Check sheet for the modelled part. Datum: model origin and axes. Units: mm. Face numbers are marked on the shaded views. A direction names the side the tool comes from. Round coordinates to 2 decimals unless told otherwise and drop trailing zeros. Order: outer loops, then holes, each group sorted by start corner. A loop starts at its lowest first (then second) coordinate and runs counter-clockwise, first axis right, second up. Notation, with made-up numbers: (36.25, 45.25) -> (49.25, 45.25) arc R19 cw to (49.25, 77.25) -> close; hole circle Ø10 at (68.25, 73). An arc over 180 degrees is marked (long way). Use CSV: the item, a comma, the result in double quotes.
```python
from build123d import *

# Parameters (mm, degrees)
SKETCH1_W           = 42
SKETCH1_H           = 25
BOSS_EXTRUDE1_DEPTH = 3
SKETCH2_W           = 42
SKETCH2_H           = 17
BOSS_EXTRUDE2_DEPTH = 6
SKETCH4_W           = 42
SKETCH4_H           = 3
BOSS_EXTRUDE4_DEPTH = 3
FILLET2_R           = 2
SKETCH5_W           = 42
SKETCH5_H           = 3
BOSS_EXTRUDE5_DEPTH = 2
SKETCH7_W           = 42
SKETCH7_H           = 3
BOSS_EXTRUDE6_DEPTH = 20
BOSS_EXTRUDE7_DEPTH = 50
BOSS_EXTRUDE8_DEPTH = 13
CUT_EXTRUDE1_DEPTH  = 13
FILLET3_R           = 10


with BuildPart() as part:
    # Sketch1 → Boss-Extrude1 (new body)
    with BuildSketch(Plane(origin=(0, 0, 0), x_dir=(1, 0, 0), z_dir=(0, 1, 0))):
        Rectangle(SKETCH1_W, SKETCH1_H)
    extrude(amount=BOSS_EXTRUDE1_DEPTH)

    # Sketch2 → Boss-Extrude2 (add)
    with BuildSketch(Plane(origin=(0, 0, 0), x_dir=(1, 0, 0), z_dir=(0, 1, 0))):
        with Locations((0, 21)):
            Rectangle(SKETCH2_W, SKETCH2_H)
    extrude(amount=BOSS_EXTRUDE2_DEPTH)

    # Sketch4 → Boss-Extrude4 (add)
    with BuildSketch(Plane(origin=(0, 0, -29.5), x_dir=(-1, 0, 0), z_dir=(0, 0, -1))):
        with Locations((0, 4.5)):
            Rectangle(SKETCH4_W, SKETCH4_H)
    extrude(amount=BOSS_EXTRUDE4_DEPTH)

    # Fillet2
    fillet2_edges = [part.edges().sort_by_distance(p)[0] for p in [
        (0, 3, -29.5),
    ]]
    fillet(fillet2_edges, radius=FILLET2_R)

    # Sketch5 → Boss-Extrude5 (add)
    with BuildSketch(Plane(origin=(0, 0, -32.5), x_dir=(-1, 0, 0), z_dir=(0, 0, -1))):
        with Locations((0, 4.5)):
            Rectangle(SKETCH5_W, SKETCH5_H)
    extrude(amount=BOSS_EXTRUDE5_DEPTH)

    # Sketch7 → Boss-Extrude6 (add)
    with BuildSketch(Plane(origin=(0, 0, -34.5), x_dir=(-1, 0, 0), z_dir=(0, 0, -1))):
        with Locations((0, 4.5)):
            Rectangle(SKETCH7_W, SKETCH7_H)
    extrude(amount=BOSS_EXTRUDE6_DEPTH)

    # Sketch6 → Boss-Extrude7 (add)
    with BuildSketch(Plane(origin=(0, 6, 0), x_dir=(1, 0, 0), z_dir=(0, 1, 0))):
        Polygon((-21, 34.5), (-1, 34.5), (-1, 54.5), (1, 54.5), (1, 34.5), (21, 34.5), (21, 32.5), (1, 32.5), (1, 12.5), (-1, 12.5), (-1, 32.5), (-21, 32.5), align=None)
    extrude(amount=BOSS_EXTRUDE7_DEPTH)

    # Sketch9 → Boss-Extrude8 (add)
    with BuildSketch(Plane(origin=(0, 6, 0), x_dir=(1, 0, 0), z_dir=(0, 1, 0))):
        Polygon((-12, 34.5), (-1, 45.5), (-1, 34.5), align=None)
        Polygon((1, 34.5), (1, 45.5), (12, 34.5), align=None)
        Polygon((12, 32.5), (1, 32.5), (1, 21.5), align=None)
        Polygon((-1, 21.5), (-1, 32.5), (-12, 32.5), align=None)
    extrude(amount=BOSS_EXTRUDE8_DEPTH)

    # Sketch10 → Cut-Extrude1 (cut)
    with BuildSketch(Plane(origin=(0, 6, 0), x_dir=(1, 0, 0), z_dir=(0, 1, 0))):
        Polygon((1, 45.5), (1, 51.581118318), (18.081118318, 34.5), (12, 34.5), align=None)
        Polygon((-1, 45.5), (-1, 51.581118318), (-18.081118318, 34.5), (-12, 34.5), align=None)
        Polygon((-12, 32.5), (-1, 21.5), (-1, 15.418881682), (-18.081118318, 32.5), align=None)
        Polygon((1, 21.5), (1, 15.418881682), (18.081118318, 32.5), (12, 32.5), align=None)
    extrude(amount=-CUT_EXTRUDE1_DEPTH, mode=Mode.SUBTRACT)

    # Fillet3
    fillet3_edges = [part.edges().sort_by_distance(p)[0] for p in [
        (21, 4.5, -54.5),
        (-21, 4.5, -54.5),
    ]]
    fillet(fillet3_edges, radius=FILLET3_R)


solid = part.part
```
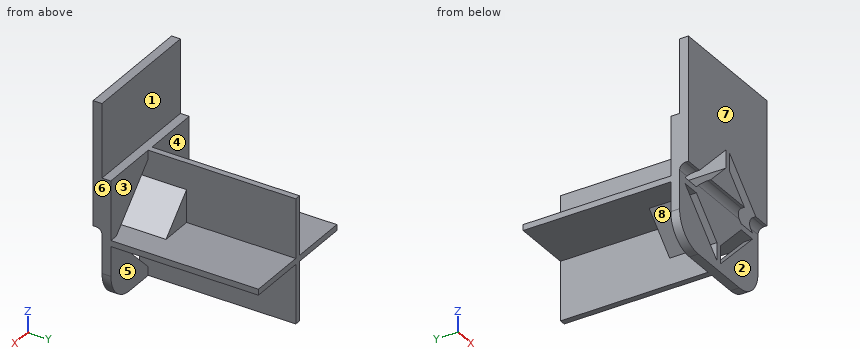
Q1. Scan lines: L1, parallel to X at y = 5, z = -16; L2, parallel to X at y = 2, z = -27.5; L3, parallel to Z at x = 4.5, y = 4. Record each from-to range of solid material in increasing order.
Result sheet:
L1,"x = -21 to -1.58, -1 to 1, 1.58 to 21"
L2,"x = -21 to -13.08, -7 to 7, 13.08 to 21"
L3,"z = -54.5 to -48.08, -42 to -25, -18.92 to -12.5"
Q2. Sectioned sample at A-A, the plane x = -6.5. Enter the section's corners in (y, z), then the cut area to 3 significant figures.
Result sheet:
outline,"(0, -29.5) -> (1, -29.5) arc R2 cw to (3, -31.5) -> (3, -40) -> (19, -40) -> (19, -34.5) -> (56, -34.5) -> (56, -32.5) -> (19, -32.5) -> (19, -27) -> (0, -27) -> close; (0, -20.92) -> (6, -20.92) -> (6, -12.5) -> (3, -12.5) -> (3, 12.5) -> (0, 12.5) -> close; (3, -54.5) -> (6, -54.5) -> (6, -46.08) -> (3, -46.08) -> close"
area,"441 mm^2"
Q3. Access from +Z, -Z, +X, -X, +Y, -Y to the whole of each face (thin tool, end or side, straight path). Record for the marked faces 1, 2, 3, 4 and 5.
Result sheet:
face 1,"+Z, +X, -X, +Y"
face 2,"-Z, +X, -X, -Y"
face 3,"+Z, +X, +Y"
face 4,"+Z, -X, +Y"
face 5,"-Z, +X, +Y"
Q4. Mould release check, pull along X, two halves, no side actions. Record for the marked faces 6, 7 and 8: pulls with the +X half, pulls with the -X half, needs draft (parallel to the pull), parting line crosses it, or undercut.
Result sheet:
face 6,"pulls with the +X half"
face 7,"needs draft"
face 8,"undercut"
Q5. Sectioned sample at B-B, the plane z = -48. Enter the section's corners in (x, y), then the cut area to 3 significant figures.
Result sheet:
outline,"(-20.37, 3) -> (-4.58, 3) -> (-4.58, 6) -> (-20.37, 6) -> close; (-1, 3) -> (1, 3) -> (1, 56) -> (-1, 56) -> close; (4.58, 3) -> (20.37, 3) -> (20.37, 6) -> (4.58, 6) -> close"
area,"201 mm^2"
Q6. Sectioned sample at D-D, the plane x = 10. Enter the section's corners in (y, z).
Result sheet:
outline,"(0, -24.42) -> (6, -24.42) -> (6, -12.5) -> (3, -12.5) -> (3, 12.5) -> (0, 12.5) -> close; (2.73, -30.5) arc R2 cw to (3, -31.5) -> (3, -36.5) -> (19, -36.5) -> (19, -34.5) -> (56, -34.5) -> (56, -32.5) -> (19, -32.5) -> (19, -30.5) -> close; (3, -54.5) -> (6, -54.5) -> (6, -42.58) -> (3, -42.58) -> close"
Q7. Go/stop test with flat-tipped pins: pin 1 (8 mm diameter, centred on x = 4, z = -2, fed in from +Y); pin 2 (3.5 mm diameter, centred on x = -4, z = -24.5, fed in from +Y); pin 3 (8 mm diameter, centred on y = 27.5, z = -6.5, fed in from +X) (3 decimals); pin 4 (1.5 mm diameter, centred on x = -6.5, y = 10.5, fed in from -Z). Record where each tip stops, or that it passes through.
Result sheet:
pin 1,"stops at y = 3"
pin 2,"stops at y = 19"
pin 3,"passes through"
pin 4,"stops at z = -40.75"
Q8. Sectioned sample at C-C, the plane y = 13.5. Enter the section's corners in (x, z).
Result sheet:
outline,"(-21, -34.5) -> (-12, -34.5) -> (-1, -45.5) -> (-1, -54.5) -> (1, -54.5) -> (1, -45.5) -> (12, -34.5) -> (21, -34.5) -> (21, -32.5) -> (12, -32.5) -> (1, -21.5) -> (1, -12.5) -> (-1, -12.5) -> (-1, -21.5) -> (-12, -32.5) -> (-21, -32.5) -> close"
